The drawing under review shows one solid part. Ordinate dimensions are in mm from its lowest x, y, z. A direction names the side the tool comes from. Coordinates: 2 decimals unless noted, no trailing zeros. Order: outer loops, then holes, each group sorted by start corner. A loop starts at its lowest first (then second) coordinate and runs counter-clockwise, first axis right, second up. Notation, with made-up numbers: (74.5, 47) -> (83.5, 47) arc R13 ccw to (83.5, 64) -> close; hole circle Ø8 at (-22.75, 78). An arc over 180 degrees is marked (long way). Write item = value, one per line.
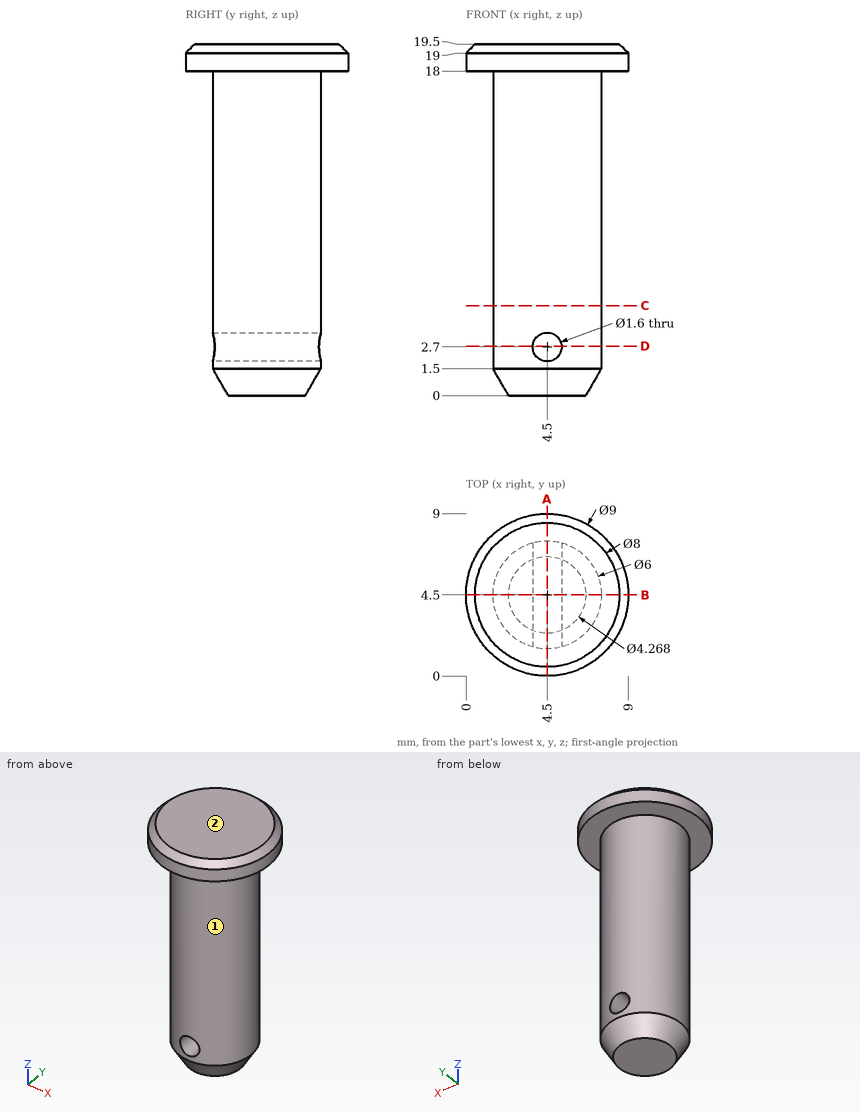
(1) We need section C-C (z = 5). Write out the cut boundary in (x, y), and give its area (3 significant figures).
Report:
outline = circle Ø6 at (4.5, 4.5)
area = 28.3 mm²
(2) We need section B-B (y = 4.5). Write out the cut boundary in (x, z), and give its area (3 significant figures).
Report:
outline = (0, 18) -> (1.5, 18) -> (1.5, 1.5) -> (2.37, 0) -> (6.63, 0) -> (7.5, 1.5) -> (7.5, 18) -> (9, 18) -> (9, 19) -> (8.5, 19.5) -> (0.5, 19.5) -> (0, 19) -> close; hole circle Ø1.6 at (4.5, 2.7)
area = 118 mm²
(3) Insertion check: pin 1 (1 mm diameter, centred on y = 7, z = 14, fed in from +X); pin 2 (4 mm diameter, centred on x = 2.5, z = 4.5, fed in from -Y); pin 3 (5 mm diameter, centred on x = 1, z = 16.5, fed in from +Y). Each pin has a flat end and moves straight along its axis. Give the tip position at first contact, or say it passes through.
Report:
pin_1 = 6.74
pin_2 = 1.5
pin_3 = 8.74
(4) For L1, parallel to Z at x = 4.5, y = 4.75; L2, parallel to Z at x = 5.5, y = 1; L3, parallel to Z at x = 5, y = 7.25 (1 decimal), list the stretches that pass through material, from the lowest coordinate up.
Report:
L1 = 0 to 1.9, 3.5 to 19.5
L2 = 18 to 19.5
L3 = 1.1 to 2.1, 3.3 to 19.5
(5) We need section D-D (z = 2.75). Write out the cut boundary in (x, y), and give its area (3 significant figures).
Report:
outline = (3.7, 1.61) -> (3.7, 7.39) arc R3 ccw to start; (5.3, 1.61) arc R3 ccw to (5.3, 7.39) -> close
area = 18.8 mm²
(6) For the marked faces 1 and 2, list the 3-axis set-ups (+Z, -Z, +X, -X, +Y, -Y) from which the entire face can be reached by the end or side of a thin tool; tool diameter is ignored.
Report:
face_1 = -Z
face_2 = +Z, +X, -X, +Y, -Y
(7) We need section A-A (x = 4.5). Write out the cut boundary in (y, z), and give its area (3 significant figures).
Report:
outline = (0, 18) -> (1.5, 18) -> (1.5, 3.5) -> (7.5, 3.5) -> (7.5, 18) -> (9, 18) -> (9, 19) -> (8.5, 19.5) -> (0.5, 19.5) -> (0, 19) -> close; (1.5, 1.5) -> (2.37, 0) -> (6.63, 0) -> (7.5, 1.5) -> (7.5, 1.9) -> (1.5, 1.9) -> close
area = 110 mm²
